Read the model definition and answer for the solid it produces. Units are mm, in the model's axes. Face numbers are marked on the shaded views. A direction names the side the tool comes from. Round coordinates to 2 decimals unless told otherwise and drop trailing zeros. Loops run counter-clockwise (first coordinate to the right, second up) from the corner with the lowest first, then second, coordinate; pieces in that order, holes last. Notation, with made-up numbers: (43.5, -37) - (86.5, -37) arc R26 cw to (86.5, -5) - close; hole circle Ø4 at (77, -16.75). An arc over 180 degrees is marked (long way). Answer as CSV lines item,"result".
```python
from build123d import *

# Parameters (mm, degrees)
BASESTEELANGLE_DEPTH = 450
TOEFILLET_R          = 10


with BuildPart() as part:
    # Sketch1 → BaseSteelAngle (new, symmetric)
    with BuildSketch(Plane.XY):
        with BuildLine():
            Line((0, 100), (0, 0))
            Line((0, 0), (100, 0))
            Line((100, 0), (100, 10))
            Line((100, 10), (22, 10))
            ThreePointArc((22, 10), (13.514718626, 13.514718626), (10, 22))
            Line((10, 22), (10, 100))
            Line((10, 100), (0, 100))
        make_face()
    extrude(amount=BASESTEELANGLE_DEPTH, both=True)

    # ToeFillet
    toefillet_edges = [part.edges().sort_by_distance(p)[0] for p in [
        (10, 100, 0),
        (100, 10, 0),
    ]]
    fillet(toefillet_edges, radius=TOEFILLET_R - 0.0001)  # a hair under: the kernel refuses the full size


solid = part.part
```
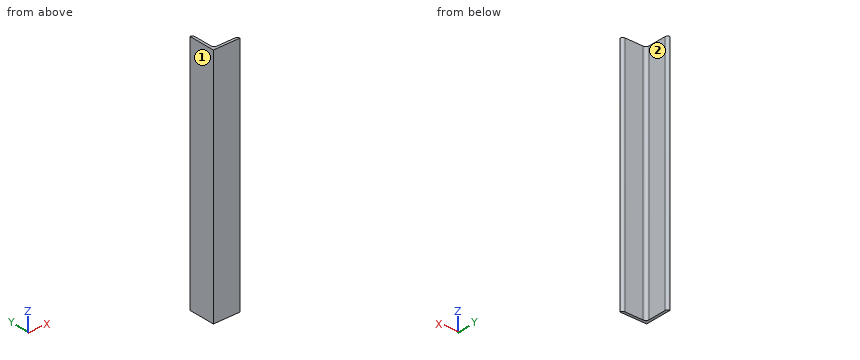
1) A cutting plane is placed at B-B, the plane x = 81. Determine the outline of the cut face in (y, z).
Entries:
outline,"(0, -450) - (10, -450) - (10, 450) - (0, 450) - close"
2) Each of these flat-tipped pins is pushed along its axis until it touches: P1, Ø10, axis at x = 35, z = -353.5, coming from the +Y side; P2, Ø1.5, axis at x = 12.5, z = -322.5, coming from the +Y side; P3, Ø6, axis at y = 73.5, z = 89, coming from the +X side. Where does it stop, or does it pass through?
Entries:
P1,"stops at y = 10"
P2,"stops at y = 15.76"
P3,"stops at x = 10"
3) A tool of negligible diameter and unlimited length cuts with its end or side. For the marked faces 1 and 2, from which of +Z, -Z, +X, -X, +Y, -Y can it reach the whole face along a straight path? Write none if from no direction.
Entries:
face 1,"+Z, -Z, -X, +Y, -Y"
face 2,"+Z, -Z, +X, +Y"
4) Find the intervals of material crossed by line 1 (Y direction, x = 53, z = 322); line 2 (X direction, y = 19, z = 68.5), in increasing order.
Entries:
line 1,"y = 0 to 10"
line 2,"x = 0 to 10.38"
